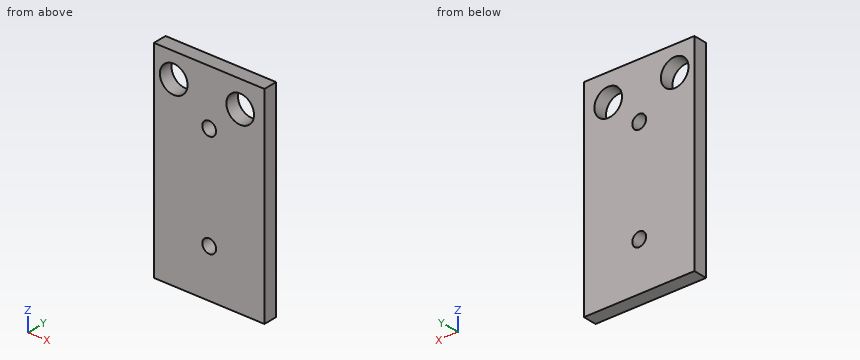
```python
from build123d import *

# Parameters (mm, degrees)
F0_W     = 101.6
F0_H     = 177.8
F1_DEPTH = 12.7
F2_W     = 101.6
F2_H     = 12.7
F3_DEPTH = 12.7
F4_R     = 12.7
F4_R_2   = 6.35
F5_DEPTH = 12.701
F6_R     = 6.35
F7_DEPTH = 12.701


# Not quite as in the source:
# - a feature names something its author has since deleted; it is built from what else it names


with BuildPart() as f1:
    # F0 (on Front) → F1 (new body)
    with BuildSketch(Plane.XZ):
        Rectangle(F0_W, F0_H)
    extrude(amount=F1_DEPTH)

    # F2 (on face) → F3 (join)
    with BuildSketch(Plane(origin=(0, 0, -88.9), x_dir=(1, 0, 0), z_dir=(0, 0, -1))):
        with Locations((0, 6.35)):
            Rectangle(F2_W, F2_H)
    extrude(amount=F3_DEPTH)

    # F4 (on face) → F5 (cut, through all)
    with BuildSketch(Plane(origin=(0, 0, 0), x_dir=(-1, 0, 0), z_dir=(0, 1, 0))):
        with Locations((-28.5075195134, 64.3249601126)):
            Circle(F4_R)
        with Locations((0, 38.1)):
            Circle(F4_R_2)
        with Locations((32.6408334076, 66.04)):
            Circle(F4_R)
    extrude(amount=-F5_DEPTH, mode=Mode.SUBTRACT)

    # F6 (on face) → F7 (cut, through all)
    with BuildSketch(Plane(origin=(0, 0, 0), x_dir=(-1, 0, 0), z_dir=(0, 1, 0))):
        with Locations((0, -57.15)):
            Circle(F6_R)
    extrude(amount=-F7_DEPTH, mode=Mode.SUBTRACT)


solid = f1.part
```
Input: part model. Units: mm. Frame: model coordinates. Round coordinates to 2 decimals unless told otherwise and drop trailing zeros. Order: outer loops, then holes, each group sorted by start corner. A loop starts at its lowest first (then second) coordinate and runs counter-clockwise, first axis right, second up. Notation, with made-up numbers: (76.25, 42) - (81.25, 42) arc R21 ccw to (81.25, 58) - close; hole circle Ø6 at (57.25, -27). An arc over 180 degrees is marked (long way). One line per question, with ' | ' between items. Start each with the question number.
1) Ray query, probe 1 along Z at (x, y) = (0, -4.75); probe 2 along Z at (x, y) = (5.5, -9.75); probe 3 along X at (y, z) = (-2, 37.5). Return the intervals inside material, ascending.
2) Cut plane B-B, the plane z = -57.15. Return the cut outline in (x, y).
3) Cut plane C-C, the plane x = 22.5. Return the cut outline in (y, z), then the cut area to 3 significant figures.
4) Cut plane D-D, the plane y = -2. Return the cut outline in (x, z), then the cut area to 3 significant figures.
5) Cut plane A-A, the plane x = 0. Return the cut outline in (y, z), then the cut area to 3 significant figures.
Worked out:
1) probe 1: z = -101.6 to -63.5, -50.8 to 31.75, 44.45 to 88.9 | probe 2: z = -101.6 to -60.32, -53.98 to 34.93, 41.27 to 88.9 | probe 3: x = -50.8 to -6.32, 6.32 to 50.8
2) outline: (-50.8, -12.7) - (-6.35, -12.7) - (-6.35, 0) - (-50.8, 0) - close; (6.35, -12.7) - (50.8, -12.7) - (50.8, 0) - (6.35, 0) - close
3) outline: (-12.7, -101.6) - (0, -101.6) - (0, 53.14) - (-12.7, 53.14) - close; (-12.7, 75.51) - (0, 75.51) - (0, 88.9) - (-12.7, 88.9) - close | area: 2,140 mm^2
4) outline: (-50.8, -101.6) - (50.8, -101.6) - (50.8, 88.9) - (-50.8, 88.9) - close; hole circle Ø25.4 at (-32.64, 66.04); hole circle Ø12.7 at (0, -57.15); hole circle Ø12.7 at (0, 38.1); hole circle Ø25.4 at (28.51, 64.32) | area: 18,100 mm^2
5) outline: (-12.7, -101.6) - (0, -101.6) - (0, -63.5) - (-12.7, -63.5) - close; (-12.7, -50.8) - (0, -50.8) - (0, 31.75) - (-12.7, 31.75) - close; (-12.7, 44.45) - (0, 44.45) - (0, 88.9) - (-12.7, 88.9) - close | area: 2,100 mm^2
